Design review of the part built by this model. Coordinates are the model's own, in mm. Face numbers are marked on the shaded views. A direction names the side the tool comes from. Give positions to 0.01 mm unless a question says otherwise; leave off trailing zeros. Write each loop counter-clockwise with the first axis right and the second up, starting at its lowest first coordinate (ties: lowest second). Pieces come first, ordered by that corner, then holes. Notation, with made-up numbers: M 29.25,13.25 L 34.25,13.25 A23 cw 34.25,27.25 Z; hole C -3,45.25 d7. An arc over 180 degrees is marked long. Use one line per item in the form item = value. Start each with the question number.
from build123d import *

# Parameters (mm, degrees)
F1_DEPTH = 76.2
F3_DEPTH = 38.101


# Not quite as in the source:
# - a feature names something its author has since deleted; it is built from what else it names


with BuildPart() as f1:
    # F0 (on Front) → F1 (new body)
    with BuildSketch(Plane.XZ):
        Polygon((0, 3.175), (0, 0), (38.1, 0), (38.1, 38.1), (34.925, 38.1), (34.925, 3.175), align=None)
    extrude(amount=F1_DEPTH)

    # F2 (on face) → F3 (cut, through all)
    with BuildSketch(Plane.XY.offset(38.1)):
        Polygon((34.925, -41.275), (34.925, 0), (0, 0), (0, -76.2), align=None)
        Polygon((38.1, 0), (34.925, 0), (34.925, -41.275), (38.1, -38.1), align=None)
    extrude(amount=-F3_DEPTH, mode=Mode.SUBTRACT)


solid = f1.part
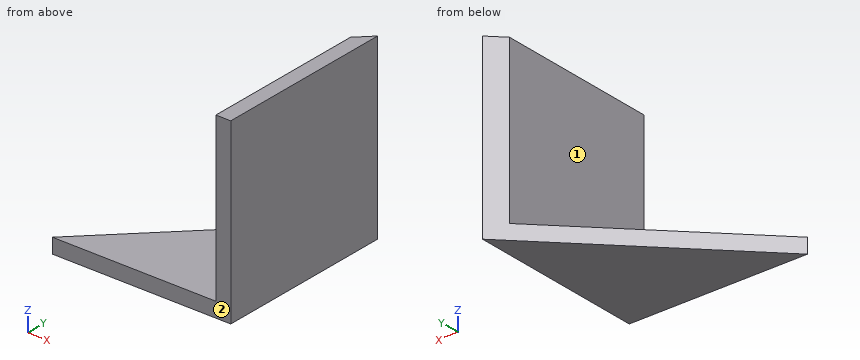
1. For the marked faces 1 and 2, list the 3-axis set-ups (+Z, -Z, +X, -X, +Y, -Y) from which the entire face can be reached by the end or side of a thin tool; tool diameter is ignored.
2. To check wall thickness, follow L1, parallel to X at y = -66, z = 12 (3 decimals); L2, parallel to Z at x = 24, y = -53 (3 decimals); L3, parallel to Y at x = 36, z = 28.5. State the ranges of each line that lie inside material, in increasing order.
3. We need section C-C (x = 19). State the section outline as (y, z) points (3 decimals).
4. We need section B-B (z = 2). State the section outline as (x, y) points.
5. Clearance check with flat-ended pins moving along their axes: pin 1 Ø17.5 at (x, y) = (9.5, -51.5) entering from +Z; pin 2 Ø3 at (y, z) = (-47, 19) entering from -X (3 decimals); pin 3 Ø12 at (x, y) = (29.5, -69.5) entering from +Z; pin 4 Ø12 at (x, y) = (23, -66.5) entering from +Z (3 decimals). State where each tip first meets the part, or that it passes through.
6. We need section D-D (y = -65). State the section outline as (x, z) points (3 decimals).
7. We need section A-A (y = -44.5). State the section outline as (x, z) points (3 decimals), and give its area (3 significant figures).
Answer block:
q1.face_1 = +Z, -X, +Y, -Y
q1.face_2 = +Z, -Z, +X, -X, -Y
q2.L1 = 34.925 to 38.1
q2.L2 = 0 to 3.175
q2.L3 = -76.2 to -40.2
q3.outline = M -76.2,0 L -57.2,0 L -57.2,3.175 L -76.2,3.175 Z
q4.outline = M 0,-76.2 L 38.1,-76.2 L 38.1,-38.1 Z
q5.pin_1 = through
q5.pin_2 = 34.925
q5.pin_3 = 38.1
q5.pin_4 = 3.175
q6.outline = M 11.2,0 L 38.1,0 L 38.1,38.1 L 34.925,38.1 L 34.925,3.175 L 11.2,3.175 Z
q7.outline = M 31.7,0 L 38.1,0 L 38.1,38.1 L 34.925,38.1 L 34.925,3.175 L 31.7,3.175 Z
q7.area = 131 mm^2
